Part model, mm, in its own coordinate system. Face numbers are marked on the shaded views. Coordinates: 2 decimals unless noted, no trailing zeros. Loops run counter-clockwise (first coordinate to the right, second up) from the corner with the lowest first, then second, coordinate; pieces in that order, holes last. Notation, with made-up numbers: M 59,41 L 67,41 A30 cw 67,79 Z; hole C -12,-24.5 d3. An arc over 180 degrees is marked long. Use a Markdown table: item, result. Add a question column.
1) Band-saw the part on C-C (z = 0.25). List the corners of the cut face in (x, y), plus the area to 3 significant figures.
2) Band-saw the part on A-A (y = 2.1). List the corners of the cut face in (x, z), plus the area to 3 significant figures.
3) Pin check, flat tips, straight feed: pin 1 Ø3 at (y, z) = (1, 2.5) entering from +X; pin 2 Ø1 at (x, y) = (-1, 4) entering from +Z. Stop position of each tip, or through.
4) Band-saw the part on D-D (z = 2.5). List the corners of the cut face in (x, y).
5) Wall check: probe 1 along X at (y, z) = (2.75, 1); probe 2 along X at (y, z) = (1.95, 0). Give the ranges that are in metal, low to high. Write a range as from..to.
6) Band-saw the part on B-B (x = 0). List the corners of the cut face in (y, z), plus the area to 3 significant figures.
7) Pull direction X, two halves, no side cores. Call the marked faces 1 and 2: released by +X, released by -X, zero draft, split by the parting line, or undercut.
from build123d import *

# Parameters (mm, degrees)
SKETCH1_R           = 1.5
BOSS_EXTRUDE1_DEPTH = 5.08


with BuildPart() as part:
    # Sketch1 → Boss-Extrude1 (new body)
    with BuildSketch(Plane(origin=(0, 0, 0), x_dir=(1, 0, 0), z_dir=(0, 1, 0))):
        Polygon((-3.922137091, -3.697862909), (3.697862909, -3.922137091), (3.922137091, 3.697862909), (-3.697862909, 3.922137091), align=None)
        Circle(SKETCH1_R, mode=Mode.SUBTRACT)
    extrude(amount=BOSS_EXTRUDE1_DEPTH)


solid = part.part
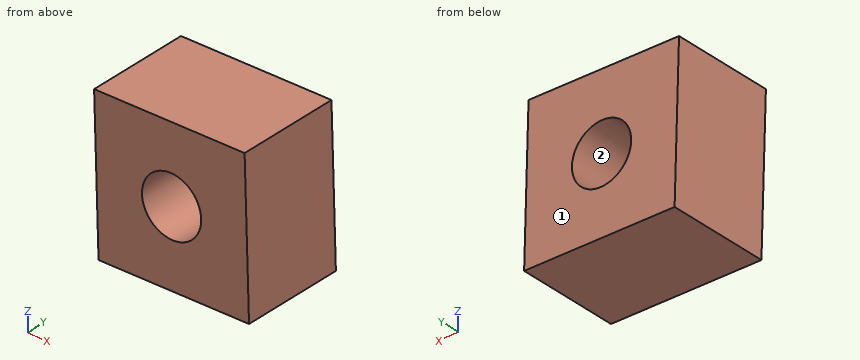
Entries:
| question | item | result |
|---|---|---|
| 1 | outline | M -3.82,0 L -1.48,0 L -1.48,5.08 L -3.82,5.08 Z; M 1.48,0 L 3.81,0 L 3.81,5.08 L 1.48,5.08 Z |
| 1 | area | 23.7 mm2 |
| 2 | outline | M -3.92,3.7 L -3.7,-3.92 L 3.92,-3.7 L 3.7,3.92 Z; hole C 0,0 d3 |
| 2 | area | 51.0 mm2 |
| 3 | pin 1 | x = 3.78 |
| 3 | pin 2 | z = 3.8 |
| 4 | outline | M -3.89,0 L 3.74,0 L 3.74,5.08 L -3.89,5.08 Z |
| 5 | probe 1 | -3.84..-1.12, 1.12..3.78 |
| 5 | probe 2 | -3.81..-1.5, 1.5..3.81 |
| 6 | outline | M 0,-3.81 L 5.08,-3.81 L 5.08,-1.5 L 0,-1.5 Z; M 0,1.5 L 5.08,1.5 L 5.08,3.81 L 0,3.81 Z |
| 6 | area | 23.5 mm2 |
| 7 | face 1 | zero draft |
| 7 | face 2 | undercut |
